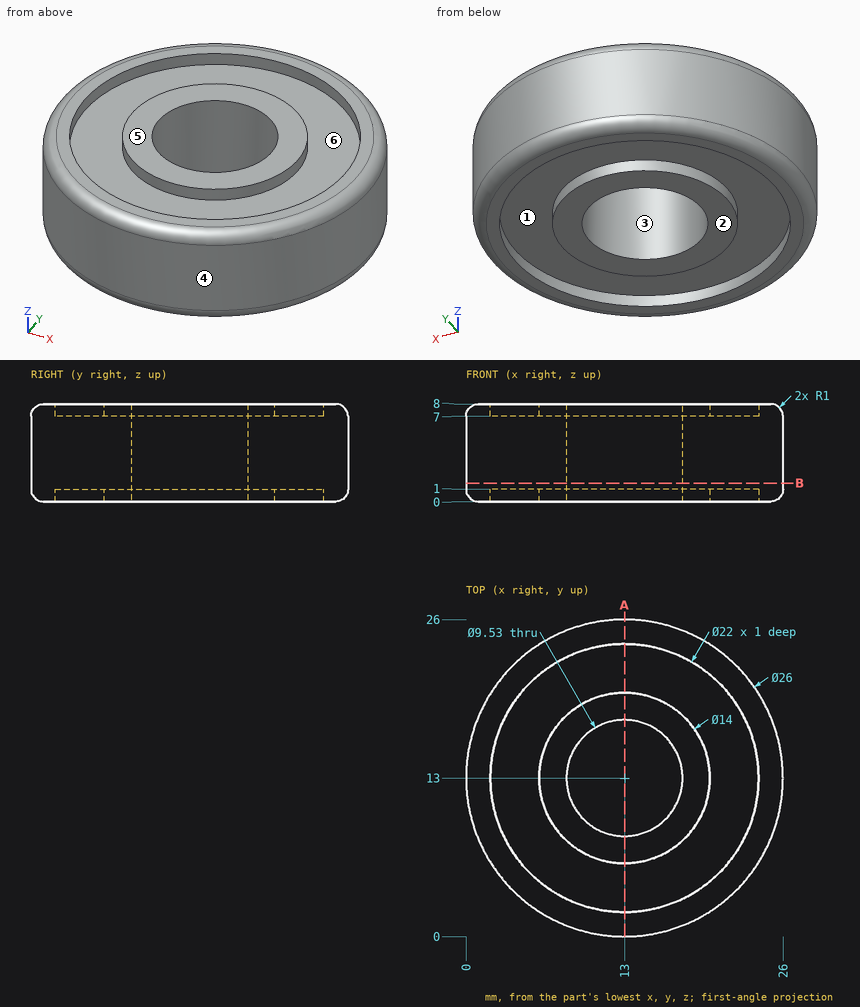
Job drawing, mm, ordinate dimensions from the low corner. One solid piece. A direction names the side the tool comes from. Give positions to 0.01 mm unless a question says otherwise; leave off trailing zeros. Order: outer loops, then holes, each group sorted by start corner. A loop starts at its lowest first (then second) coordinate and runs counter-clockwise, first axis right, second up. Notation, with made-up numbers: (30, -7) - (59, -7) arc R10 ccw to (59, 7) - close; hole circle Ø8 at (-5.5, -4.5). An arc over 180 degrees is marked (long way). Return JSON: item names as keys, results as strings.
1) Probe line 1 (Y direction, x = 13, z = 5.5) (3 decimals); line 2 (Y direction, x = 13, z = 7.7) (3 decimals); line 3 (X direction, y = 8, z = 4). List the from-to ranges inside material, lowest first. Write a range as from..to.
Geometry says:
{"line 1": "0..8.235, 17.765..26", "line 2": "0.286..2, 6..8.235, 17.765..20, 24..25.714", "line 3": "1..25"}
2) Cut at B-B, the plane z = 1.5. Give the cut face in (x, y) (3 decimals).
Geometry says:
{"outline": "circle Ø26 at (13, 13); hole circle Ø9.53 at (13, 13)"}
3) Pull direction Y, two halves, no side cores. Call the marked faces 1, 2, 3 and 4: pulls with the +Y half, pulls with the -Y half, needs draft (parallel to the pull), parting line crosses it, or undercut.
Geometry says:
{"face 1": "undercut", "face 2": "needs draft", "face 3": "undercut", "face 4": "parting line crosses it"}
4) Cut at A-A, the plane x = 13. Give the cut face in (y, z) (3 decimals).
Geometry says:
{"outline": "(0, 1) arc R1 ccw to (1, 0) - (2, 0) - (2, 1) - (6, 1) - (6, 0) - (8.235, 0) - (8.235, 8) - (6, 8) - (6, 7) - (2, 7) - (2, 8) - (1, 8) arc R1 ccw to (0, 7) - close; (17.765, 0) - (20, 0) - (20, 1) - (24, 1) - (24, 0) - (25, 0) arc R1 ccw to (26, 1) - (26, 7) arc R1 ccw to (25, 8) - (24, 8) - (24, 7) - (20, 7) - (20, 8) - (17.765, 8) - close"}
5) Flat gauge pins, fed straight in: P1, Ø4, axis at y = 21, z = 7, coming from the +X side; P2, Ø1, axis at y = 4, z = 3.5, coming from the +X side; P3, Ø5.5, axis at x = 13, y = 13, coming from the +Z side; P4, Ø1, axis at y = 20, z = 3, coming from the +X side. Where does each tip first touch, or does it go through?
Geometry says:
{"P1": "x = 24.53", "P2": "x = 22.84", "P3": "through", "P4": "x = 24.26"}
6) 3-axis set-ups, long thin cutter, end or side, ignore diameter. For the marked faces 5 and 6: which of +Z, -Z, +X, -X, +Y, -Y reach the whole face in a straight line?
Geometry says:
{"face 5": "+Z, +X, -X, +Y, -Y", "face 6": "+Z"}
